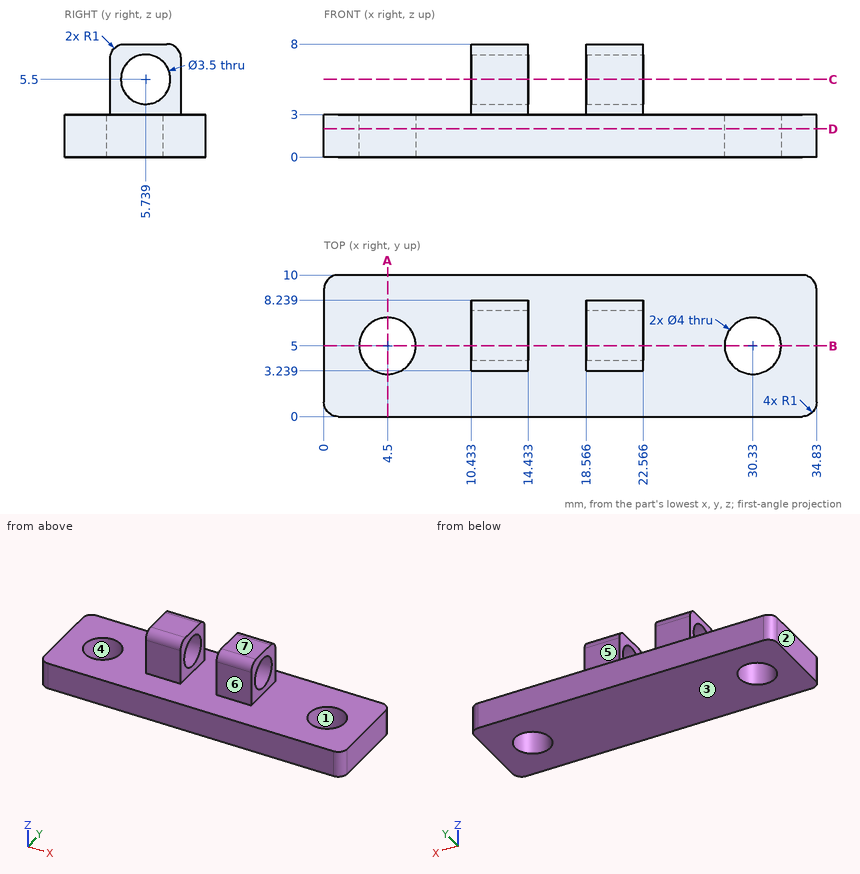
Study the drawing (mm; zero at the part's minimum x, y, z) and answer. A direction names the side the tool comes from. Round coordinates to 2 decimals unless told otherwise and drop trailing zeros. Loops run counter-clockwise (first coordinate to the right, second up) from the corner with the lowest first, then second, coordinate; pieces in that order, holes last. Notation, with made-up numbers: (88.5, -10) -> (99.5, -10) arc R14 ccw to (99.5, 5) -> close; hole circle Ø11 at (88, -34). An arc over 180 degrees is marked (long way). One line per item, written item: value.
1) A cutting plane is placed at A-A (x = 4.5). Determine the outline of the cut face in (y, z).
Answer list:
outline: (0, 0) -> (3, 0) -> (3, 3) -> (0, 3) -> close; (7, 0) -> (10, 0) -> (10, 3) -> (7, 3) -> close
2) A cutting plane is placed at B-B (y = 5). Determine the outline of the cut face in (x, z).
Answer list:
outline: (0, 0) -> (2.5, 0) -> (2.5, 3) -> (0, 3) -> close; (6.5, 0) -> (28.33, 0) -> (28.33, 3) -> (22.57, 3) -> (22.57, 3.91) -> (18.57, 3.91) -> (18.57, 3) -> (14.43, 3) -> (14.43, 3.91) -> (10.43, 3.91) -> (10.43, 3) -> (6.5, 3) -> close; (10.43, 7.09) -> (14.43, 7.09) -> (14.43, 8) -> (10.43, 8) -> close; (18.57, 7.09) -> (22.57, 7.09) -> (22.57, 8) -> (18.57, 8) -> close; (32.33, 0) -> (34.83, 0) -> (34.83, 3) -> (32.33, 3) -> close
3) A cutting plane is placed at C-C (z = 5.5). Determine the outline of the cut face in (x, y).
Answer list:
outline: (10.43, 3.24) -> (14.43, 3.24) -> (14.43, 3.99) -> (10.43, 3.99) -> close; (10.43, 7.49) -> (14.43, 7.49) -> (14.43, 8.24) -> (10.43, 8.24) -> close; (18.57, 3.24) -> (22.57, 3.24) -> (22.57, 3.99) -> (18.57, 3.99) -> close; (18.57, 7.49) -> (22.57, 7.49) -> (22.57, 8.24) -> (18.57, 8.24) -> close
4) For the marked faces 5, 6 and 7, determine the directions among +Z, -Z, +X, -X, +Y, -Y from which every point of the face is accessible in a straight line to the end or side of a thin tool.
Answer list:
face 5: +Z, +X, -X, +Y
face 6: +Z, +X, -X, -Y
face 7: +Z, +X, -X, +Y, -Y
5) A cutting plane is placed at D-D (z = 2). Determine the outline of the cut face in (x, y), and give its area (3 significant figures).
Answer list:
outline: (0, 1) arc R1 ccw to (1, 0) -> (33.83, 0) arc R1 ccw to (34.83, 1) -> (34.83, 9) arc R1 ccw to (33.83, 10) -> (1, 10) arc R1 ccw to (0, 9) -> close; hole circle Ø4 at (4.5, 5); hole circle Ø4 at (30.33, 5)
area: 322 mm²
6) The mould has two halves that part along X. Classify the marked faces 1, 2, 3 and 4: pulls with the +X half, pulls with the -X half, needs draft (parallel to the pull), parting line crosses it, or undercut.
Answer list:
face 1: undercut
face 2: pulls with the -X half
face 3: needs draft
face 4: undercut
7) Flat-ended cylindrical pins translate along their axes: P1, Ø4, axis at y = 5.74, z = 5.5, coming from the +X side; P2, Ø1.2, axis at x = 20, z = 5.5, coming from the +Y side; P3, Ø3, axis at x = 4.5, y = 5, coming from the -Z side; P4, Ø1.5, axis at y = 5, z = 4.5, coming from the -X side. Find the tip coordinate at first contact, or state that the pin passes through.
Answer list:
P1: stops at x = 22.57
P2: stops at y = 8.24
P3: passes through
P4: stops at x = 10.43
8) Consider L1, parallel to X at y = 4.5, z = 7; L2, parallel to X at y = 6, z = 0.5; L3, parallel to Y at x = 4.5, z = 1.3. Determine where each line is inside the solid, lowest interval first. Write a range as [from, to].
Answer list:
L1: x = [10.43, 14.43], [18.57, 22.57]
L2: x = [0, 2.77], [6.23, 28.6], [32.06, 34.83]
L3: y = [0, 3], [7, 10]
